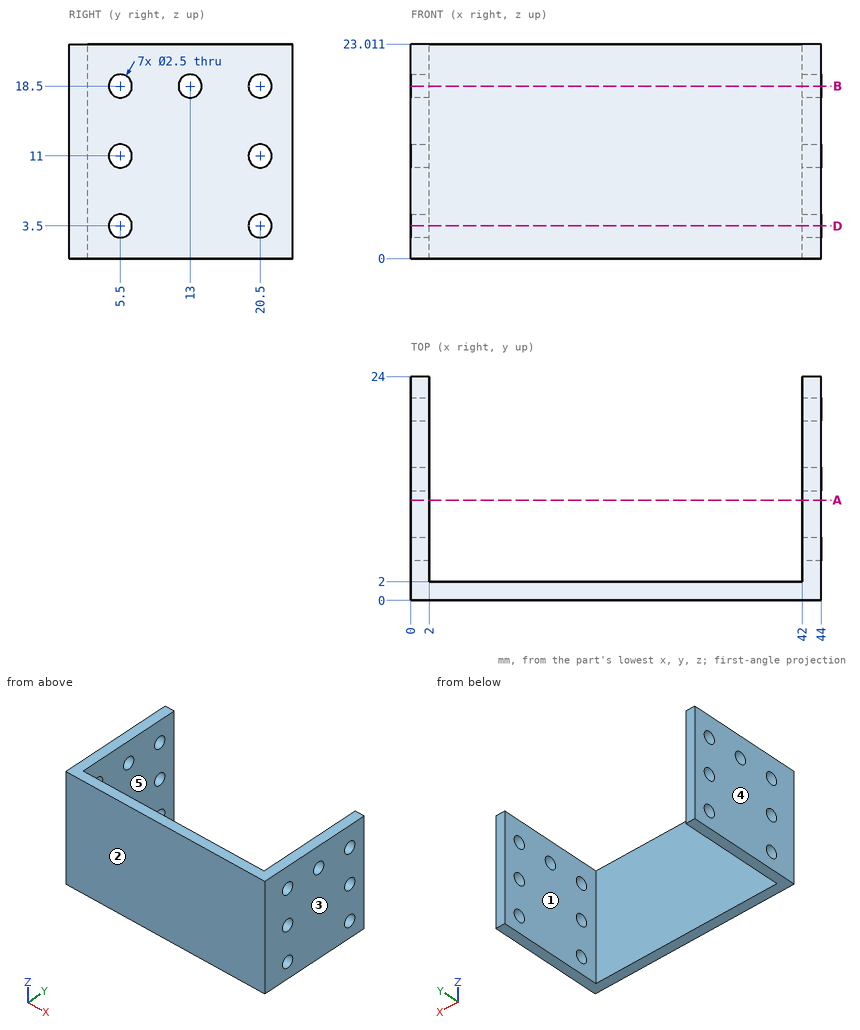
The figure shows three views and two pictorial views of one solid part (mm, origin at its lowest corner). Answer the questions. A direction names the side the tool comes from. Give positions to 0.01 mm unless a question says otherwise; leave off trailing zeros. Write each loop counter-clockwise with the first axis right and the second up, starting at its lowest first coordinate (ties: lowest second). Pieces come first, ordered by that corner, then holes. Notation, with made-up numbers: (25, 35) - (41, 35) arc R24 ccw to (41, 74) - close; hole circle Ø10 at (68, -24). An arc over 180 degrees is marked (long way). Use one line per item in the form item = value. Start each with the question number.
1) Find section B-B on z = 18.5. Count the separate pieces of the cut face and the enclosed holes in it, plus the area to 3 significant figures.
2) A tool of negligible diameter and unlimited length cuts with its end or side. For the marked faces 4 and 5, from which of +Z, -Z, +X, -X, +Y, -Y can it reach the whole face along a straight path? Write none if from no direction.
3) The mould has two halves that part along X. Classify the marked faces 1, 2 and 3: pulls with the +X half, pulls with the -X half, needs draft (parallel to the pull), parting line crosses it, or undercut.
4) Consider line 1 along Z through (x, y) = (0.85, 5.5); line 2 along Y through (x, z) = (1.1, 11); line 3 along X through (y, z) = (9.5, 21). Determine where each line is inside the solid, lowest interval first. Write a range as from..to.
5) Find section D-D on z = 3.5. Determine the outline of the cut face in (x, y), plus the area to 3 significant figures.
6) Flat-ended cylindrical pins translate along their axes: pin 1 Ø1.5 at (y, z) = (5.5, 3.5) entering from -X; pin 2 Ø10 at (x, z) = (15.5, 3.5) entering from +Y. Find the tip coordinate at first contact, or state that the pin passes through.
7) Find section A-A on y = 10.75. Determine the outline of the cut face in (x, z).
Geometry results:
q1.separate_pieces = 7
q1.enclosed_holes = 0
q1.area = 146 mm2
q2.face_4 = +Z, -Z, -X, +Y, -Y
q2.face_5 = +Z, -Z, +Y
q3.face_1 = undercut
q3.face_2 = needs draft
q3.face_3 = pulls with the +X half
q4.line_1 = 0..2.25, 4.75..9.75, 12.25..17.25, 19.75..23.01
q4.line_2 = 0..4.25, 6.75..19.25, 21.75..24
q4.line_3 = 0..2, 42..44
q5.outline = (0, 0) - (44, 0) - (44, 4.25) - (42, 4.25) - (42, 2) - (2, 2) - (2, 4.25) - (0, 4.25) - close; (0, 6.75) - (2, 6.75) - (2, 19.25) - (0, 19.25) - close; (0, 21.75) - (2, 21.75) - (2, 24) - (0, 24) - close; (42, 6.75) - (44, 6.75) - (44, 19.25) - (42, 19.25) - close; (42, 21.75) - (44, 21.75) - (44, 24) - (42, 24) - close
q5.area = 156 mm2
q6.pin_1 = through
q6.pin_2 = 2
q7.outline = (0, 0) - (2, 0) - (2, 23.01) - (0, 23.01) - close; (42, 0) - (44, 0) - (44, 23.01) - (42, 23.01) - close
